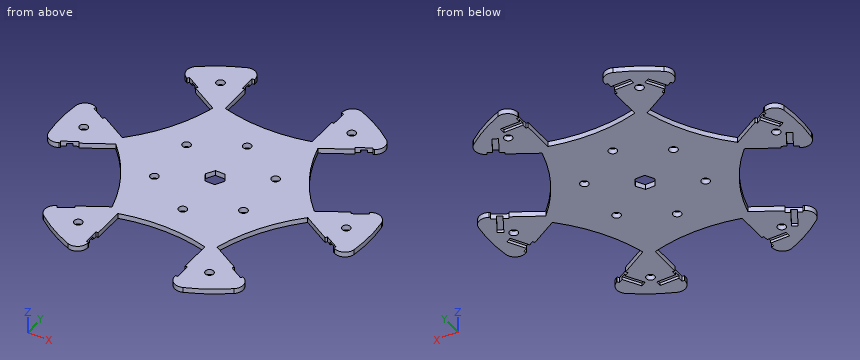
```python
from build123d import *

# Parameters (mm, degrees)
SKETCH3_R                = 60.062756644
DISK_DEPTH               = 2
SKETCH4_W                = 50.4
SKETCH4_H                = 2.2
AXLE_DEPTH               = 1.1
ROLLER_DEPTH             = 2
WASHER_DEPTH             = 2
FILLET1_R                = 4
CIRPATTERN1_COUNT        = 6
FILLET1_OF_CIRPATTERN1_R = 4
SKETCH9_R                = 1.6
ROLLER_SCREW_DEPTH       = 2
CIRPATTERN3_COUNT        = 6
HEX_AXLE_REACH           = 4
SKETCH11_R               = 1.6
HUB_SCREWS_DEPTH         = 2
CIRPATTERN4_COUNT        = 6


with BuildPart() as part:
    # Sketch3 → Disk (new body)
    with BuildSketch(Plane.XY):
        Circle(SKETCH3_R)
    extrude(amount=DISK_DEPTH)

    # Sketch4 → Axle (cut)
    with BuildSketch(Plane.XY):
        with Locations((0, 48.55177146)):
            Rectangle(SKETCH4_W, SKETCH4_H)
    axle = extrude(amount=AXLE_DEPTH, mode=Mode.SUBTRACT)

    # Sketch7 → Roller (cut)
    with BuildSketch(Plane.XY):
        with BuildLine():
            Line((16.912362698, 62.893833964), (-16.912362698, 62.893833964))
            Line((-16.912362698, 62.893833964), (-16.912362698, 33.342312944))
            ThreePointArc((-16.912362698, 33.342312944), (0, 31.103542919), (16.912362698, 33.342312944))
            Line((16.912362698, 33.342312944), (16.912362698, 62.893833964))
        make_face()
    roller = extrude(amount=ROLLER_DEPTH, mode=Mode.SUBTRACT)

    # Sketch8 → Washer (cut)
    with BuildSketch(Plane.XY):
        Polygon((-17.812362698, 51.55177146), (-16.912362698, 51.55177146), (-16.412362698, 51.55177146), (-16.412362698, 45.55177146), (-16.912362698, 45.55177146), (-17.812362698, 45.55177146), align=None)
        Polygon((17.812362698, 51.55177146), (17.812362698, 45.55177146), (16.912362698, 45.55177146), (16.412362698, 45.55177146), (16.412362698, 51.55177146), (16.912362698, 51.55177146), align=None)
    washer = extrude(amount=WASHER_DEPTH, mode=Mode.SUBTRACT)

    # Fillet1
    fillet1_edges = [part.edges().sort_by_distance(p)[0] for p in [
        (-16.912362698, 57.632514466, 1),
        (16.912362698, 57.632514466, 1),
    ]]
    fillet(fillet1_edges, radius=FILLET1_R)

    # CirPattern1: Axle, Roller, Washer ×6 about axis
    cirpattern1_axis = Axis((0, 0, 0), (0, 0, 1))
    for i in range(1, CIRPATTERN1_COUNT):
        add(axle.rotate(cirpattern1_axis, i * 360 / CIRPATTERN1_COUNT), mode=Mode.SUBTRACT)
        add(roller.rotate(cirpattern1_axis, i * 360 / CIRPATTERN1_COUNT), mode=Mode.SUBTRACT)
        add(washer.rotate(cirpattern1_axis, i * 360 / CIRPATTERN1_COUNT), mode=Mode.SUBTRACT)

    # Fillet1 of CirPattern1
    fillet1_of_cirpattern1_edges = [part.edges().sort_by_distance(p)[0] for p in [
        (-58.36740296, 14.169721499, 1),
        (-41.455040262, 43.462792967, 1),
        (-41.455040262, -43.462792967, 1),
        (-58.36740296, -14.169721499, 1),
        (16.912362698, -57.632514466, 1),
        (-16.912362698, -57.632514466, 1),
        (58.36740296, -14.169721499, 1),
        (41.455040262, -43.462792967, 1),
        (41.455040262, 43.462792967, 1),
        (58.36740296, 14.169721499, 1),
    ]]
    fillet(fillet1_of_cirpattern1_edges, radius=FILLET1_OF_CIRPATTERN1_R)

    # Sketch9 → Roller screw (cut)
    with BuildSketch(Plane.XY.offset(2)):
        with Locations((-25.531378322, -44.221644441)):
            Circle(SKETCH9_R)
    roller_screw = extrude(amount=-ROLLER_SCREW_DEPTH, mode=Mode.SUBTRACT)

    # CirPattern3: Roller screw ×6 about axis
    cirpattern3_axis = Axis((0, 0, 0), (0, 0, 1))
    for i in range(1, CIRPATTERN3_COUNT):
        add(roller_screw.rotate(cirpattern3_axis, i * 360 / CIRPATTERN3_COUNT), mode=Mode.SUBTRACT)

    # Sketch10 → Hex axle (cut, up to next)
    with BuildSketch(Plane.XY, mode=Mode.PRIVATE) as hex_axle_sk1:
        Polygon((3.781644263, 0), (1.890822132, 3.275), (-1.890822132, 3.275), (-3.781644263, 0), (-1.890822132, -3.275), (1.890822132, -3.275), align=None)
    hex_axle_tool1 = extrude(hex_axle_sk1.sketch, amount=HEX_AXLE_REACH, mode=Mode.PRIVATE) & part.part
    add(hex_axle_tool1.solids().sort_by_distance((0, 0, 0))[0], mode=Mode.SUBTRACT)

    # Sketch11 → Hub screws (cut)
    with BuildSketch(Plane.XY):
        with Locations((0, 20)):
            Circle(SKETCH11_R)
    hub_screws = extrude(amount=HUB_SCREWS_DEPTH, mode=Mode.SUBTRACT)

    # CirPattern4: Hub screws ×6 about axis
    cirpattern4_axis = Axis((0, 0, 0), (0, 0, 1))
    for i in range(1, CIRPATTERN4_COUNT):
        add(hub_screws.rotate(cirpattern4_axis, i * 360 / CIRPATTERN4_COUNT), mode=Mode.SUBTRACT)


solid = part.part
```
Geometry: final body of the model. Coordinates: model frame, mm. Coordinates: 2 decimals unless noted, no trailing zeros. Write each loop counter-clockwise with the first axis right and the second up, starting at its lowest first coordinate (ties: lowest second). Pieces come first, ordered by that corner, then holes. Notation, with made-up numbers: M -9,72.5 L -4,72.5 A22 ccw -4,110.5 Z; hole C 44.5,-26 d8. An arc over 180 degrees is marked long. Use CSV: the item, a comma, the result in double quotes. Start each with the question number.
1. Cut plane C-C on x = -43. Return the cut outline in (y, z), plus the area to 3 significant figures.
2. Ray query, probe 1 along X at (y, z) = (-9.5, 1.15); probe 2 along Y at (x, z) = (16.5, 0.7); probe 3 along Y at (x, z) = (-38, 0.2). Return the intervals inside material, ascending.
3. Cut plane D-D on x = 41.5. Return the cut outline in (y, z).
4. First-contact query: P1, Ø0.6, axis at x = 0, z = 1, coming from the -Y side; P2, Ø1.2, axis at x = -22.5, z = 0.5, coming from the +Y side; P3, Ø0.7, axis at x = 22, y = -48.5, coming from the -Z side. Flat tips, straight axial feed; report the tip coordinate or a pass-through.
5. Cut plane B-B on y = -20. Return the cut outline in (x, z), plus the area to 3 significant figures.
6. Cut plane A-A on x = 0. Return the cut outline in (y, z) (3 decimals).
Entries:
1,outline,"M -5.3,0 L 5.3,0 L 5.3,2 L -5.3,2 Z"
1,area,"21.2 mm²"
2,probe 1,"-59.17 to -52.08, -30.89 to -18.84, -15.8 to 15.8, 18.84 to 30.89, 52.08 to 59.17"
2,probe 2,"-33.23 to -11.37, -8.63 to 8.63, 11.37 to 33.23"
2,probe 3,"-46.21 to -42.03, -2.41 to 2.41, 42.03 to 46.21"
3,outline,"M -4.43,0 L 4.43,0 L 4.43,2 L -4.43,2 Z"
4,P1,"y = -31.1"
4,P2,"y = 55.89"
4,P3,"z = 1.1"
5,outline,"M -24.59,0 L -1.6,0 L -1.6,2 L -24.59,2 Z; M 1.6,0 L 24.59,0 L 24.59,2 L 1.6,2 Z"
5,area,"92.0 mm²"
6,outline,"M -31.104,0 L -21.6,0 L -21.6,2 L -31.104,2 Z; M -18.4,0 L -3.275,0 L -3.275,2 L -18.4,2 Z; M 3.275,0 L 18.4,0 L 18.4,2 L 3.275,2 Z; M 21.6,0 L 31.104,0 L 31.104,2 L 21.6,2 Z"
